For this review, take the finished solid that the model builds, in its own axes (mm). A direction names the side the tool comes from. Coordinates: 2 decimals unless noted, no trailing zeros. Loops run counter-clockwise (first coordinate to the right, second up) from the corner with the lowest first, then second, coordinate; pieces in that order, holes last. Notation, with made-up numbers: M 29,-1.75 L 82,-1.75 A5 ccw 82,4.25 Z; hole C 76,-20.75 d1. An arc over 180 degrees is marked long. Answer as a JSON object with one key per item and string values. Group by question number.
Item 1: Add section B-B (y = 4.5). State the section outline as (x, z) points (3 decimals).
Item 2: Mouldability with a two-part tool opening along X and no side actions: class faces 1 (the face through (-2.7, 12.3, 0)), 2 (the face through (0.1, 16.65, 2.5)), 3 (the face through (-2.925, 3.944, -5.161)) as +X half, -X half, draft (parallel to the pull), parting line (faces both ways), or undercut.
Item 3: Add section D-D (z = 3). State the section outline as (x, y) points.
Item 4: Wall thickness on L1, parallel to X at y = 6.75, z = 0; L2, parallel to Z at x = 1, y = 6.25; L3, parallel to Z at x = -2, y = 10: over which ranges is each line inside the solid? List them lowest first. Write a range as from..to.
Item 5: Add section A-A (z = 0). State the section outline as (x, y) points.
Item 6: Tool access review of faces 4 (the face through (-3.5, 12.3, -4.5)), 5 (the face through (3.01, 3.94, -5.11)): name each direction out of +Z, -Z, +X, -X, +Y, -Y from which nothing blocks a thin tool from reaching the whole face with its end or side.
Item 7: Insertion check: pin 1 (2.5 mm diameter, centred on x = 0, z = 0, fed in from +Y); pin 2 (4.5 mm diameter, centred on x = 0, y = 13, fed in from -Z); pin 3 (6 mm diameter, centred on x = -3.5, y = 14.5, fed in from +Z); pin 4 (1.5 mm diameter, centred on x = 0.5, y = 7, fed in from +Z). Each pin has a flat end and moves straight along its axis. Give the tip position at first contact, or say it passes through.
Item 8: Add section C-C (x = 1.25). State the section outline as (y, z) points.
from build123d import *

# Parameters (mm, degrees)
SKETCH_1_R      = 1.6
EXTRUDE_1_DEPTH = 8
SKETCH_2_R      = 5.7
EXTRUDE_2_DEPTH = 8.65


with BuildPart() as part:
    # 草图1 → 凸台-拉伸1 (new body)
    with BuildSketch(Plane(origin=(0, 0, 0), x_dir=(1, 0, 0), z_dir=(0, 1, 0))):
        Polygon((0, 6.85), (-5.932274016, 3.425), (-5.932274016, -3.425), (0, -6.85), (5.932274016, -3.425), (5.932274016, 3.425), align=None)
        with Locations(Location((0, 0, 0), (0, 0, 270))):
            Circle(SKETCH_1_R, mode=Mode.SUBTRACT)
    extrude(amount=EXTRUDE_1_DEPTH)

    # 草图2 → 凸台-拉伸2 (add)
    with BuildSketch(Plane(origin=(0, 8, 0), x_dir=(1, 0, 0), z_dir=(0, 1, 0))):
        with Locations(Location((0, 0, 0), (0, 0, 270))):
            Circle(SKETCH_2_R)
        with BuildLine():
            Line((-1.966596044, 1.85), (1.966596044, 1.85))
            ThreePointArc((1.966596044, 1.85), (2.7, 0), (1.966596044, -1.85))
            Line((1.966596044, -1.85), (-1.966596044, -1.85))
            ThreePointArc((-1.966596044, -1.85), (-2.7, 0), (-1.966596044, 1.85))
        make_face(mode=Mode.SUBTRACT)
    extrude(amount=EXTRUDE_2_DEPTH)


solid = part.part
From the geometry:
{
 "1": {"outline": "M -5.932,-3.425 L 0,-6.85 L 5.932,-3.425 L 5.932,3.425 L 0,6.85 L -5.932,3.425 Z; hole C 0,0 d3.2"},
 "2": {"face 1": "undercut", "face 2": "draft", "face 3": "-X half"},
 "3": {"outline": "M -5.93,0 L 5.93,0 L 5.93,8 L 4.85,8 L 4.85,16.65 L -4.85,16.65 L -4.85,8 L -5.93,8 Z"},
 "4": {"L1": "x = -5.93..-1.6, 1.6..5.93", "L2": "z = -6.27..-1.25, 1.25..6.27", "L3": "z = -5.34..-1.81, 1.81..5.34"},
 "5": {"outline": "M -5.93,0 L -1.6,0 L -1.6,8 L -2.7,8 L -2.7,16.65 L -5.7,16.65 L -5.7,8 L -5.93,8 Z; M 1.6,0 L 5.93,0 L 5.93,8 L 5.7,8 L 5.7,16.65 L 2.7,16.65 L 2.7,8 L 1.6,8 Z"},
 "6": {"face 4": "+Y", "face 5": "-Z, +X, +Y, -Y"},
 "7": {"pin 1": "passes through", "pin 2": "stops at z = -5.7", "pin 3": "stops at z = 5.68", "pin 4": "stops at z = 6.85"},
 "8": {"outline": "M 0,-6.13 L 8,-6.13 L 8,-5.56 L 16.65,-5.56 L 16.65,-1.85 L 8,-1.85 L 8,-1 L 0,-1 Z; M 0,1 L 8,1 L 8,1.85 L 16.65,1.85 L 16.65,5.56 L 8,5.56 L 8,6.13 L 0,6.13 Z"}
}
